Job drawing, mm, ordinate dimensions from the low corner. One solid piece. Give positions to 0.01 mm unless a question says otherwise; leave off trailing zeros. Write each loop counter-clockwise with the first axis right and the second up, starting at its lowest first coordinate (ties: lowest second). Pieces come first, ordered by that corner, then holes. Notation, with made-up numbers: (45.5, 73.25) - (52.5, 73.25) arc R25 ccw to (52.5, 102.25) - close; hole circle Ø5 at (61.5, 86.5). An arc over 180 degrees is marked (long way). Answer as a JSON object with one key per item and string values.
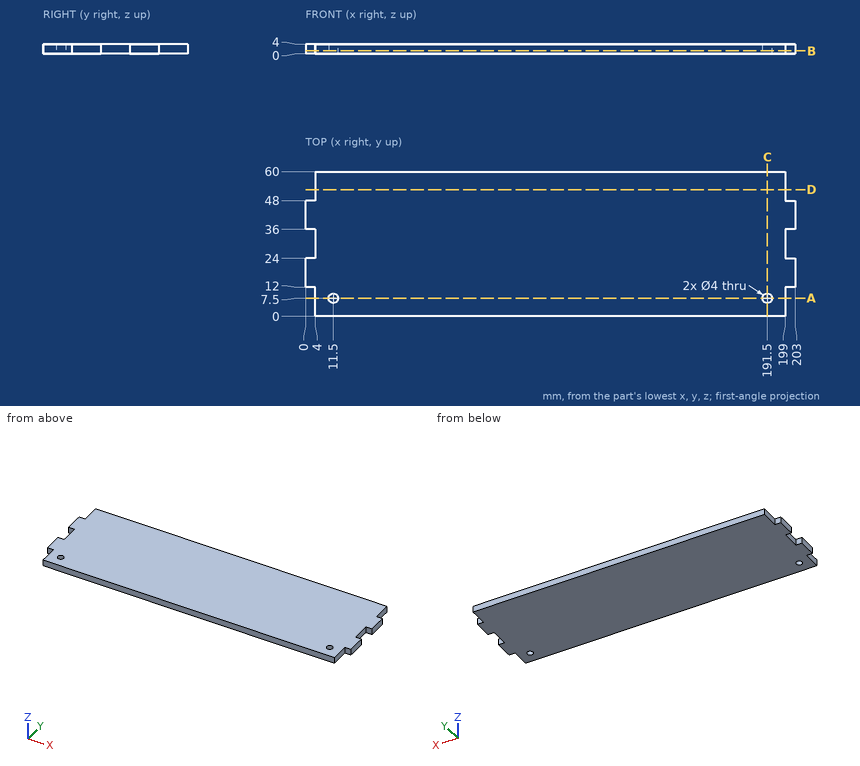
Item 1: Flat gauge pins, fed straight in: P1, Ø2, axis at x = 66.5, y = 34, coming from the -Z side; P2, Ø1.2, axis at y = 7, z = 2, coming from the +X side; P3, Ø2, axis at x = 201.5, z = 3, coming from the +Y side; P4, Ø1.2, axis at x = 200.5, z = 1.5, coming from the -Y side. Where does each tip first touch, or does it go through?
Entries:
{"P1": "z = 0", "P2": "x = 199", "P3": "y = 48", "P4": "y = 12"}
Item 2: Cut at A-A (y = 7.5). Give the cut face in (x, z), and give its area (3 significant figures).
Entries:
{"outline": "(4, 0) - (9.5, 0) - (9.5, 4) - (4, 4) - close; (13.5, 0) - (189.5, 0) - (189.5, 4) - (13.5, 4) - close; (193.5, 0) - (199, 0) - (199, 4) - (193.5, 4) - close", "area": "748 mm2"}
Item 3: Cut at B-B (z = 1.1). Give the cut face in (x, y), and give its area (3 significant figures).
Entries:
{"outline": "(0, 12) - (4, 12) - (4, 0) - (199, 0) - (199, 12) - (203, 12) - (203, 24) - (199, 24) - (199, 36) - (203, 36) - (203, 48) - (199, 48) - (199, 60) - (4, 60) - (4, 48) - (0, 48) - (0, 36) - (4, 36) - (4, 24) - (0, 24) - close; hole circle Ø4 at (11.5, 7.5); hole circle Ø4 at (191.5, 7.5)", "area": "11,900 mm2"}
Item 4: Probe line 1 (X direction, y = 7.5, z = 1.2); line 2 (Y direction, x = 11.5, z = 2); line 3 (X direction, y = 54, z = 2.45). List the from-to ranges inside material, lowest first. Write a range as from..to.
Entries:
{"line 1": "4..9.5, 13.5..189.5, 193.5..199", "line 2": "0..5.5, 9.5..60", "line 3": "4..199"}
Item 5: Cut at C-C (x = 191.5). Give the cut face in (y, z), and give its area (3 significant figures).
Entries:
{"outline": "(0, 0) - (5.5, 0) - (5.5, 4) - (0, 4) - close; (9.5, 0) - (60, 0) - (60, 4) - (9.5, 4) - close", "area": "224 mm2"}
Item 6: Cut at D-D (y = 52.5). Give the cut face in (x, z), and give its area (3 significant figures).
Entries:
{"outline": "(4, 0) - (199, 0) - (199, 4) - (4, 4) - close", "area": "780 mm2"}
